Autodesk Inventor part; units mm, degrees
ref_plane "YZ Plane" through (0, 0, 0) normal (1, 0, 0) x (0, 1, 0)
ref_plane "XZ Plane" through (0, 0, 0) normal (0, 1, 0) x (-1, 0, 0)
ref_plane "XY Plane" through (0, 0, 0) normal (0, 0, 1) x (1, 0, 0)
sketch "Sketch1" plane through (0, 0, 0) normal (0, 0, 1) x (1, 0, 0)
  line L0 (2, 0) -> (65, 0)
  line L1 (65, 0) -> (65, 29)
  line L2 (65, 29) -> (2, 29)
  line L3 (0, 27) -> (0, 2)
  arc A0 (2, 29) -> (0, 27) centre (2, 27) ccw
  arc A1 (0, 2) -> (2, 0) centre (2, 2) ccw
  line L4 (20, 29) -> (20, 0)
  line L5 (55, 29) -> (55, 0)
  circle A2 centre (7, 24.5) radius 1.5
  circle A3 centre (7, 4.5) radius 1.5
  circle A4 centre (13.5, 24.5) radius 1.5
  circle A5 centre (13.5, 4.5) radius 1.5
  line L6 (65, 0) -> (65, -2.5)
  line L7 (65, -2.5) -> (55, -2.5)
  line L8 (55, -2.5) -> (55, 0)
  line L9 (55, 29) -> (55, 31.5)
  line L10 (55, 31.5) -> (65, 31.5)
  line L11 (65, 31.5) -> (65, 29)
  point P0 (0, 0)
  point P1 (0, 29)
  dimension "d0" = 65
  dimension "d1" = 29
  dimension "d2" = 2
  dimension "d3" = 20
  dimension "d4" = 10
  dimension "d5" = 3
  dimension "d6" = 3
  dimension "d7" = 4.5
  dimension "d8" = 4.5
  dimension "d9" = 20
  dimension "d10" = 3
  dimension "d11" = 3
  dimension "d12" = 20
  dimension "d13" = 6.5
  dimension "d14" = 7
  dimension "d24" = 2.5
  dimension "d25" = 2.5
extrude "Extrusion1" add sketch "Sketch1" along normal blind 5 contours L4 L2 L5 L0
extrude "Extrusion2" add sketch "Sketch1" along normal blind 7 contours A1 L3 A0 L2 L4 L0
extrude "Extrusion3" add sketch "Sketch1" along normal blind 26.25 contours L5 L2 L1 L0
sketch "Sketch2" plane through (55, 0, 5) normal (-1, 0, 0) x (0, 0, 1)
  line L0 (21.25, 29) -> (21.25, 0)
  circle A0 centre (21.25, 14.5) radius 10
  point P0 (-5, 0)
  point P1 (21.25, 4.5)
  point P2 (21.25, 24.5)
  dimension "d21" = 20
extrude "Extrusion4" cut sketch "Sketch2" against normal blind 20 contours L0 A0 picked at (15.0351, 13.318)
extrude "Extrusion5" add sketch "Sketch1" along normal blind 26.25 contours L0 L6 L7 L8 | L9 L10 L11 L2
chamfer "Chamfer1" distance 2.5 angle 45 1 edges at (55, 0, 2.5)
chamfer "Chamfer2" distance 2.5 angle 45 1 edges at (55, 29, 2.5)
chamfer "Chamfer4" distance 0.6 angle 45 6 edges at (20, 14.5, 7) (11, 0, 7) (0.5858, 0.5858, 7) (0, 14.5, 7) (0.5858, 28.4142, 7) (11, 29, 7)
sketch "Sketch5" plane through (55, 14.5, 26.25) normal (-1, 0, 0) x (0, 0, 1)
  circle A0 centre (-15, 0) radius 2.05
  line L0 (0, -10) -> (0, -17)
  point P0 (-26.25, -14.5)
  dimension "d48" = 4.1
  dimension "d49" = 15
extrude "Extrusion7" cut sketch "Sketch5" against normal blind 26.25
extrude "Extrusion8" cut sketch "Sketch5" along normal blind 26.25
sketch "Sketch6" plane through (55, 14.5, 26.25) normal (-1, 0, 0) x (0, 0, 1)
  line L0 (0, 17) -> (0, 10)
  line L1 (-21.25, -17) -> (0, -17)
  line L2 (0, 17) -> (-8.8131, 17)
  line L3 (-8.8131, 17) -> (-8.8131, -17)
  line L4 (-8.8131, -17) -> (0, -17)
  line L5 (0, -17) -> (0, 17)
  point P0 (-26.25, -14.5)
  point P1 (-15.25, -17)
extrude "Extrusion9" cut sketch "Sketch6" against normal blind 26.25
chamfer "Chamfer5" distance 3 angle 45 1 edges at (55, 14.5, 5)
equation "\"BendRadius\" = Thickness"
equation "\"BendReliefWidth\" = Thickness"
equation "\"BendReliefDepth\" = 0.5 * Thickness"
equation "\"CornerReliefSize\" = 4 * Thickness"
equation "\"MinimumRemnant\" = 2 * Thickness"
equation "\"TransitionRadius\" = BendRadius"
equation "\"JacobiRadiusSize\" = BendRadius"
equation "\"GapSize\" = Thickness"
properties part number "tool4_2"
Part model, mm, in its own coordinate system. A direction names the side the tool comes from. Coordinates: 2 decimals unless noted, no trailing zeros. Write each loop counter-clockwise with the first axis right and the second up, starting at its lowest first coordinate (ties: lowest second). Pieces come first, ordered by that corner, then holes. Notation, with made-up numbers: (88, -10.5) - (145, -10.5) arc R32 cw to (145, 27.5) - close; hole circle Ø11 at (-9, 10.5). An arc over 180 degrees is marked (long way). Put each result on its own line as item: value.
1. Band-saw the part on D-D (z = 11.25). Write the cut outline in (x, y), then the cut area to 3 significant figures.
Final values:
outline: (55, -2.5) - (65, -2.5) - (65, 12.45) - (55, 12.45) - close; (55, 16.55) - (65, 16.55) - (65, 31.5) - (55, 31.5) - close
area: 299 mm²
2. Band-saw the part on C-C (x = 7). Write the cut outline in (y, z), then the cut area to 3 significant figures.
Final values:
outline: (0, 0) - (3, 0) - (3, 7) - (0.6, 7) - (0, 6.4) - close; (6, 0) - (23, 0) - (23, 7) - (6, 7) - close; (26, 0) - (29, 0) - (29, 6.4) - (28.4, 7) - (26, 7) - close
area: 161 mm²
3. Flat gauge pins, fed straight in: pin 1 Ø5.5 at (x, y) = (11, 8.5) entering from +Z; pin 2 Ø1.8 at (x, y) = (7, 24.5) entering from -Z; pin 3 Ø5 at (x, z) = (19.5, 2.5) entering from +Y; pin 4 Ø1 at (x, y) = (46, 12.5) entering from +Z. Where does each tip first touch, or does it go through?
Final values:
pin 1: stops at z = 7
pin 2: passes through
pin 3: stops at y = 29
pin 4: stops at z = 5
4. Band-saw the part on A-A (y = 24.5). Write the cut outline in (x, z).
Final values:
outline: (0, 0) - (5.5, 0) - (5.5, 7) - (0.6, 7) - (0, 6.4) - close; (8.5, 0) - (12, 0) - (12, 7) - (8.5, 7) - close; (15, 0) - (65, 0) - (65, 17.44) - (55, 17.44) - (55, 8) - (52, 5) - (20, 5) - (20, 6.4) - (19.4, 7) - (15, 7) - close
5. 3-axis set-ups, long thin cutter, end or side, ignore diameter. For faces 5 (the flat face through (20, 15, 6)), 6 (the flat face through (10, 15, 7)), 7 (the conical face through (0.85, 0.83, 6.76)): which of +Z, -Z, +X, -X, +Y, -Y reach the whole face in a straight line?
Final values:
face 5: +Z, +Y, -Y
face 6: +Z, -X, +Y, -Y
face 7: +Z, -X, -Y
6. Band-saw the part on B-B (z = 1.75). Give the number of separate pieces and of enclosed holes in the cut face, then the cut area to 3 significant figures.
Final values:
separate pieces: 1
enclosed holes: 4
area: 1,910 mm²
7. Two-plate mould, pull along X, no slides. Class faces 1 (the conical face through (0.83, 28.15, 6.76)), 2 (the flat face through (27, 0, 2)), 3 (the cylindrical face through (5.5, 4.43, 3.45)), 4 (the flat face through (65, 14, 9)): +X half, -X half, draft (parallel to the pull), parting line (faces both ways), or undercut.
Final values:
face 1: -X half
face 2: draft
face 3: undercut
face 4: +X half
8. Probe line 1 along Y through (x, z) = (7, 2.5); line 2 along Y through (x, z) = (58, 11.5); line 3 along X through (y, z) = (5, 1.5). List the from-to ranges inside material, lowest first. Write a range as [from, to].
Final values:
line 1: y = [0, 3], [6, 23], [26, 29]
line 2: y = [-2.5, 12.47], [16.53, 31.5]
line 3: x = [0, 5.59], [8.41, 12.09], [14.91, 65]
